```python
from build123d import *

# Parameters (mm, degrees)
F0_R        = 19.05
F1_DEPTH    = 254
F2_T        = -0.635
F3_W        = 10.16
F3_H        = 50.8
F3_H_2      = 127
F4_DEPTH    = 38.1
F5_T1_DEPTH = 127.6645661416
F5_T3_DEPTH = 127.6553906563
F5_T5_DEPTH = 127.6553906563
F5_T7_DEPTH = 127.6645661416


# Not quite as in the source:
# - a fillet or chamfer that OpenCascade refuses, or shapes differently, is made with other operations: its cross-section is extruded or revolved along the edge and cut away or added


with BuildPart() as f1:
    # F0 (on Top) → F1 (new body)
    with BuildSketch(Plane.XY):
        Circle(F0_R)
    extrude(amount=F1_DEPTH)

    # F2
    f2_openings = [f1.faces().sort_by_distance(p)[0] for p in [
        (0, 0, 0),
        (0, 0, 254),
    ]]
    offset(amount=F2_T, openings=f2_openings)

    # F3 (on Front) → F4 (cut, symmetric)
    with BuildSketch(Plane.XZ):
        with Locations((0, 50.8)):
            Rectangle(F3_W, F3_H)
        with Locations((-3.17e-08, 114.3)):
            Rectangle(F3_W, F3_H)
        with Locations((-0.4444076066, 213.36)):
            Rectangle(F3_W, F3_H_2)
    extrude(amount=F4_DEPTH, both=True, mode=Mode.SUBTRACT)

    # F5: fillet of radius 25.4 on 4 edges, made by hand

    # F5_s2 → F5_t1 (cut)
    with BuildSketch(Plane.XZ.offset(-45.9331805498)):
        with BuildLine():
            ThreePointArc((-5.5244076066, 228.6), (-12.9638953644, 246.5605122421), (-30.9244076066, 254))
            Line((-30.9244076066, 254), (-5.5244076066, 254))
            Line((-5.5244076066, 254), (-5.5244076066, 228.6))
        make_face()
    extrude(amount=F5_T1_DEPTH, mode=Mode.SUBTRACT)

    # F5_s4 → F5_t3 (cut)
    with BuildSketch(Plane.XZ.offset(-45.6780049332)):
        with BuildLine():
            ThreePointArc((30.0355923934, 254), (12.0750801513, 246.5605122421), (4.6355923934, 228.6))
            Line((4.6355923934, 228.6), (4.6355923934, 254))
            Line((4.6355923934, 254), (30.0355923934, 254))
        make_face()
    extrude(amount=F5_T3_DEPTH, mode=Mode.SUBTRACT)

    # F5_s6 → F5_t5 (cut)
    with BuildSketch(Plane.XZ.offset(-81.9773857231)):
        with BuildLine():
            ThreePointArc((30.0355923934, 254), (12.0750801513, 246.5605122421), (4.6355923934, 228.6))
            Line((4.6355923934, 228.6), (4.6355923934, 254))
            Line((4.6355923934, 254), (30.0355923934, 254))
        make_face()
    extrude(amount=F5_T5_DEPTH, mode=Mode.SUBTRACT)

    # F5_s8 → F5_t7 (cut)
    with BuildSketch(Plane.XZ.offset(-81.7313855918)):
        with BuildLine():
            ThreePointArc((-30.9244076066, 254), (-12.9638953644, 246.5605122421), (-5.5244076066, 228.6))
            Line((-5.5244076066, 228.6), (-5.5244076066, 254))
            Line((-5.5244076066, 254), (-30.9244076066, 254))
        make_face()
    extrude(amount=F5_T7_DEPTH, mode=Mode.SUBTRACT)


solid = f1.part
```
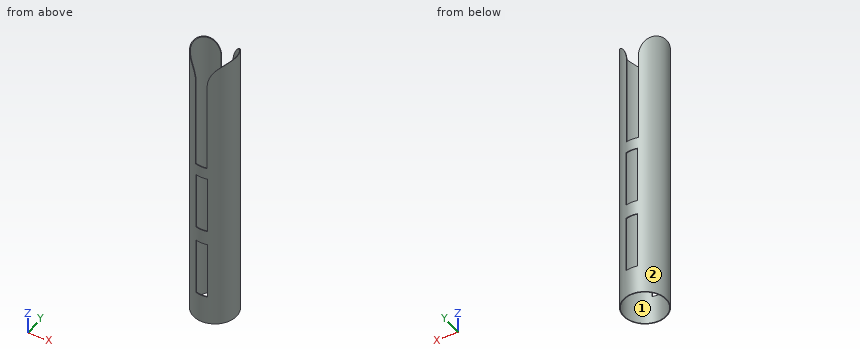
Source: CAD feature listing. Evaluate the final solid. Frame: model axes, mm. Face numbers are marked on the shaded views. Coordinates: 2 decimals unless noted, no trailing zeros. Loops run counter-clockwise (first coordinate to the right, second up) from the corner with the lowest first, then second, coordinate; pieces in that order, holes last. Notation, with made-up numbers: M -9.75,48.25 L 36.25,48.25 A15 ccw 36.25,65.25 Z; hole C 34,85 d11. An arc over 180 degrees is marked long. Use CSV: the item, a comma, the result in double quotes.
(1) Line query: line 1 (X direction, y = 0, z = 133.5) (3 decimals); line 2 (Y direction, x = -9.5, z = 129.5); line 3 (Y direction, x = 12, z = 97.5). Output: solid intervals per line, ascending. Write a range as [from, to].
Answers follow:
line 1,"[-19.05, -18.415], [18.415, 19.05]"
line 2,"[-16.51, -15.78], [15.78, 16.51]"
line 3,"[-14.8, -13.97], [13.97, 14.8]"
(2) Contact query for flat-ended pins moving along their axis: pin 1 (6 mm diameter, centred on x = -8.5, z = 93, fed in from -Y); pin 2 (1.2 mm diameter, centred on x = 0, y = -18.5, fed in from +Z); pin 3 (4 mm diameter, centred on x = -6.5, z = 179.5, fed in from +Y). Output: stop coordinate, or through.
Answers follow:
pin 1,"y = -18.24"
pin 2,"z = 149.86"
pin 3,"y = 18.23"
(3) Cut plane A-A on z = 125.5. Return loops of the section in (x, y) (3 decimals).
Answers follow:
outline,"M -5.08,-18.36 L -5.08,-17.7 A18.415 cw -5.08,17.7 L -5.08,18.36 A19.05 ccw Z; M 5.08,-18.36 A19.05 ccw 5.08,18.36 L 5.08,17.7 A18.415 cw 5.08,-17.7 Z"
(4) Cut plane C-C on y = 0. Return loops of the section in (x, z) (3 decimals).
Answers follow:
outline,"M -19.05,0 L -18.415,0 L -18.415,250.706 A25.4 ccw -19.05,251.053 Z; M 18.415,0 L 19.05,0 L 19.05,251.501 A25.4 ccw 18.415,251.186 Z"
(5) Draft query along X for the marked faces 1 and 2. Return one class per face: pulls with the +X half, pulls with the -X half, needs draft (parallel to the pull), parting line crosses it, or undercut.
Answers follow:
face 1,"undercut"
face 2,"parting line crosses it"
(6) Cut plane B-B on x = 0. Return loops of the section in (y, z) (3 decimals).
Answers follow:
outline,"M -19.05,0 L -18.415,0 L -18.415,25.4 L -19.05,25.4 Z; M -19.05,76.2 L -18.415,76.2 L -18.415,88.9 L -19.05,88.9 Z; M -19.05,139.7 L -18.415,139.7 L -18.415,149.86 L -19.05,149.86 Z; M 18.415,0 L 19.05,0 L 19.05,25.4 L 18.415,25.4 Z; M 18.415,76.2 L 19.05,76.2 L 19.05,88.9 L 18.415,88.9 Z; M 18.415,139.7 L 19.05,139.7 L 19.05,149.86 L 18.415,149.86 Z"
